from build123d import *

# Parameters (mm, degrees)
F0_R     = 7.5
F1_DEPTH = 4
F2_R     = 9.5
F3_DEPTH = 2.5
F4_R     = 2.375
F5_DEPTH = 4.001
F7_DEPTH = 2


with BuildPart() as f1:
    # F0 (on Front) → F1 (new body)
    with BuildSketch(Plane.XZ):
        with BuildLine():
            ThreePointArc((-34, -12.5), (-25.161165, -8.838835), (-21.5, 0))
            ThreePointArc((-21.5, 0), (-25.161165, 8.838835), (-34, 12.5))
            ThreePointArc((-34, 12.5), (-45.225331, 5.499267), (-43.876975, -7.66129))
            ThreePointArc((-43.876975, -7.66129), (-39.499267, -11.225331), (-34, -12.5))
        make_face()
        with Locations((-34, 0)):
            Circle(F0_R, mode=Mode.SUBTRACT)
        with BuildLine():
            ThreePointArc((-34, 12.5), (-25.161165, 8.838835), (-21.5, 0))
            ThreePointArc((-21.5, 0), (-25.161165, -8.838835), (-34, -12.5))
            Line((-34, -12.5), (34, -12.5))
            ThreePointArc((34, -12.5), (21.5, 0), (34, 12.5))
            Line((34, 12.5), (-34, 12.5))
        make_face()
        with BuildLine():
            Line((-46.247449, -12.5), (-34, -12.5))
            ThreePointArc((-34, -12.5), (-39.499267, -11.225331), (-43.876975, -7.66129))
            ThreePointArc((-43.876975, -7.66129), (-43.553369, -10.819824), (-46.247449, -12.5))
        make_face()
        Polygon((34, -12.5), (-34, -12.5), (-46.247449, -12.5), (-57.5, -12.5), (-57.5, -27.5), (57.5, -27.5), (57.5, -12.5), (46.247449, -12.5), align=None)
        with BuildLine():
            ThreePointArc((46.5, 0), (42.838835, 8.838835), (34, 12.5))
            ThreePointArc((34, 12.5), (21.5, 0), (34, -12.5))
            ThreePointArc((34, -12.5), (39.499267, -11.225331), (43.876975, -7.66129))
            ThreePointArc((43.876975, -7.66129), (45.826077, -4.048939), (46.5, 0))
        make_face()
        with Locations((34, 0)):
            Circle(F0_R, mode=Mode.SUBTRACT)
        with BuildLine():
            ThreePointArc((43.876975, -7.66129), (39.499267, -11.225331), (34, -12.5))
            Line((34, -12.5), (46.247449, -12.5))
            ThreePointArc((46.247449, -12.5), (43.553369, -10.819824), (43.876975, -7.66129))
        make_face()
    extrude(amount=F1_DEPTH)

    # F2 (on face) → F3 (cut)
    with BuildSketch(Plane.XZ.offset(4)):
        with Locations((-34, 0)):
            Circle(F2_R)
        with Locations((34, 0)):
            Circle(F2_R)
    extrude(amount=-F3_DEPTH, mode=Mode.SUBTRACT)

    # F4 (on face) → F5 (cut, through all)
    with BuildSketch(Plane.XZ.offset(4)):
        with Locations((0, -20)):
            Circle(F4_R)
        with Locations((42.155199, -20)):
            Circle(F4_R)
        with Locations((-42.155199, -20)):
            Circle(F4_R)
    extrude(amount=-F5_DEPTH, mode=Mode.SUBTRACT)

    # F6 (on face) → F7 (cut)
    with BuildSketch(Plane.XZ.offset(4)):
        Polygon((2.626944, -15.45), (-2.626944, -15.45), (-5.253887, -20), (-2.626944, -24.55), (2.626944, -24.55), (5.253887, -20), align=None)
        Polygon((-39.528255, -15.45), (-44.782142, -15.45), (-47.409086, -20), (-44.782142, -24.55), (-39.528255, -24.55), (-36.901311, -20), align=None)
        Polygon((44.782142, -15.45), (39.528255, -15.45), (36.901311, -20), (39.528255, -24.55), (44.782142, -24.55), (47.409086, -20), align=None)
    extrude(amount=-F7_DEPTH, mode=Mode.SUBTRACT)


solid = f1.part
Design review of the part built by this model. Coordinates are the model's own, in mm. A direction names the side the tool comes from. Coordinates: 2 decimals unless noted, no trailing zeros. Write each loop counter-clockwise with the first axis right and the second up, starting at its lowest first coordinate (ties: lowest second). Pieces come first, ordered by that corner, then holes. Notation, with made-up numbers: (-23, 86) - (-18, 86) arc R32 ccw to (-18, 113) - close; hole circle Ø2 at (-30.5, 31). An arc over 180 degrees is marked (long way). Use one line per item in the form item = value.
Q1. Consider section B-B (y = -3). Count the separate pieces of the cut face and the enclosed holes in it, plus the area to 3 significant figures.
Taken from the geometry:
separate_pieces = 1
enclosed_holes = 5
area = 3,160 mm^2
Q2. Consider section A-A (x = 0). Write out the cut boundary in (y, z) (3 decimals).
Taken from the geometry:
outline = (-4, -27.5) - (0, -27.5) - (0, -22.375) - (-2, -22.375) - (-2, -24.55) - (-4, -24.55) - close; (-4, -15.45) - (-2, -15.45) - (-2, -17.625) - (0, -17.625) - (0, 12.5) - (-4, 12.5) - close
Q3. The part is to be moulded in two halves that separate along Z. For faces 1 (the flat face through (-1, -2, -27.5)), 2 (the cylindrical face through (26.507, -0.74, 0.33)), 3 (the flat face through (-1, 0, -7)), say which applies: +Z half, -Z half, draft (parallel to the pull), parting line (faces both ways), or undercut.
Taken from the geometry:
face_1 = -Z half
face_2 = undercut
face_3 = draft
Q4. For probe 1 along X at (y, z) = (-1.65, 0.5); probe 2 along X at (y, z) = (-1.4, 3.5); probe 3 along X at (y, z) = (-2.55, -18), list the stretches that pass through material, from the lowest coordinate up.
Taken from the geometry:
probe_1 = -46.49 to -43.49, -24.51 to 24.51, 43.49 to 46.49
probe_2 = -46 to -40.63, -27.37 to 27.37, 40.63 to 46
probe_3 = -57.5 to -46.25, -38.06 to -4.1, 4.1 to 38.06, 46.25 to 57.5
Q5. Insertion check: pin 1 Ø12 at (x, z) = (-34, 0) entering from +Y; pin 2 Ø2 at (x, y) = (42, -2.5) entering from +Z; pin 3 Ø1.6 at (x, y) = (-42, -3) entering from +Z; pin 4 Ø2 at (y, z) = (-2, 1.5) entering from +X. Each pin has a flat end and moves straight along its axis. Give the tip position at first contact, or say it passes through.
Taken from the geometry:
pin_1 = through
pin_2 = 10.36
pin_3 = 10.22
pin_4 = 46.49
Q6. Machinability: for faces 4 (the flat face through (0, -2, 12.5)), 5 (the flat face through (-42, -3, -15.45)), which of the approach directions +Z, -Z, +X, -X, +Y, -Y give a long, thin tool a straight path to every point of the face, cutting with its end or side? Answer none if there is none.
Taken from the geometry:
face_4 = +Z, +X, -X, +Y, -Y
face_5 = -Y
